```python
from build123d import *

# Parameters (mm, degrees)
BASE_FLANGE1_DEPTH = 1220
SKETCH6_W          = 10
SKETCH6_H          = 19.2634
CUT_EXTRUDE1_DEPTH = 1350.246604201
CUT_EXTRUDE2_REACH = 1300.516
FILLET1_R          = 1


# Sheet-metal steps are written as plain solids
with BuildPart() as part:
    # Sketch1 → Base-Flange1 (new body)
    with BuildSketch(Plane(origin=(0, 0, 0), x_dir=(0, 0, -1), z_dir=(1, 0, 0))):
        with BuildLine():
            Line((-128.767123288, 0.95890411), (-128.767123288, -13.30449589))
            ThreePointArc((-128.767123288, -13.30449589), (-128.551378143, -13.825350745), (-128.030523288, -14.04109589))
            Line((-128.030523288, -14.04109589), (440.496276712, -14.04109589))
            ThreePointArc((440.496276712, -14.04109589), (441.017131567, -13.825350745), (441.232876712, -13.30449589))
            Line((441.232876712, -13.30449589), (441.232876712, 5.95890411))
            Line((441.232876712, 5.95890411), (444.232876712, 5.95890411))
            Line((444.232876712, 5.95890411), (444.232876712, -13.30449589))
            ThreePointArc((444.232876712, -13.30449589), (443.138451911, -15.946671089), (440.496276712, -17.04109589))
            Line((440.496276712, -17.04109589), (-128.030523288, -17.04109589))
            ThreePointArc((-128.030523288, -17.04109589), (-130.672698486, -15.946671089), (-131.767123288, -13.30449589))
            Line((-131.767123288, -13.30449589), (-131.767123288, 0.95890411))
            Line((-131.767123288, 0.95890411), (-128.767123288, 0.95890411))
        make_face()
    extrude(amount=BASE_FLANGE1_DEPTH)

    # Sketch6 → Cut-Extrude1 (cut, through all)
    with BuildSketch(Plane(origin=(0, 0, -444.232876712), x_dir=(-1, 0, 0), z_dir=(0, 0, -1))):
        with Locations((-1215, -3.67279589)):
            Rectangle(SKETCH6_W, SKETCH6_H)
        with Locations((-5, -3.67279589)):
            Rectangle(SKETCH6_W, SKETCH6_H)
    extrude(amount=-CUT_EXTRUDE1_DEPTH, mode=Mode.SUBTRACT)

    # Sketch8 → Cut-Extrude2 (cut, up to next)
    with BuildSketch(Plane(origin=(0, -14.04109589, 0), x_dir=(1, 0, 0), z_dir=(0, 1, 0)), mode=Mode.PRIVATE) as cut_extrude2_sk1:
        with BuildLine():
            Line((903.689592114, 440.496276712), (783.689592114, 440.496276712))
            Line((783.689592114, 440.496276712), (783.689592114, 405.496276712))
            ThreePointArc((783.689592114, 405.496276712), (785.154058208, 401.960742806), (788.689592114, 400.496276712))
            Line((788.689592114, 400.496276712), (898.689592114, 400.496276712))
            ThreePointArc((898.689592114, 400.496276712), (902.22512602, 401.960742806), (903.689592114, 405.496276712))
            Line((903.689592114, 405.496276712), (903.689592114, 440.496276712))
        make_face()
    cut_extrude2_tool1 = extrude(cut_extrude2_sk1.sketch, amount=-CUT_EXTRUDE2_REACH, mode=Mode.PRIVATE) & part.part
    add(cut_extrude2_tool1.solids().sort_by_distance((843.689592, -14.041096, -420.538583))[0], mode=Mode.SUBTRACT)

    # Fillet1
    fillet1_edges = [part.edges().sort_by_distance(p)[0] for p in [
        (610, 5.95890411, -441.232876712),
        (610, 5.95890411, -444.232876712),
    ]]
    fillet(fillet1_edges, radius=FILLET1_R)


solid = part.part
```
Geometry: final body of the model. Coordinates: model frame, mm. A direction names the side the tool comes from. Coordinates: 2 decimals unless noted, no trailing zeros. Order: outer loops, then holes, each group sorted by start corner. A loop starts at its lowest first (then second) coordinate and runs counter-clockwise, first axis right, second up. Notation, with made-up numbers: M 29,19 L 36,19 A36 ccw 36,55 Z; hole C 56,20 d5. An arc over 180 degrees is marked long. Answer in a Markdown table with one row per item. Add a question column.
Q1. Contact query for flat-ended pins moving along their axis: P1, Ø3.5, axis at x = 1216, z = 130.5, coming from the +Y side; P2, Ø1.5, axis at y = -8.5, z = -442, coming from the -X side; P3, Ø1.5, axis at x = 870, y = -16, coming from the -Z side; P4, Ø1.5, axis at y = -12.5, z = -224.5, coming from the +X side. Output: stop coordinate, or through.
Q2. Section query D-D on x = 685.5. Return the cut outline in (y, z), and give its area (3 significant figures).
Q3. Reachability of faces 1 (the flat face through (601, -14.041, -152)), 2 (the flat face through (601, -17.041, -160)) from +Z, -Z, +X, -X, +Y, -Y: full face, straight path, thin tool, end or side. Return the list, or none.
Q4. Line query: L1, parallel to Z at x = 411.5, y = -9.25; L2, parallel to Z at x = 633, y = -13.5; L3, parallel to Y at x = 1103, z = -371.5. Output: solid intervals per line, ascending.
Q5. Section query B-B on y = -6. Return the cut outline in (x, z), and give its area (3 significant figures).
Q6. Section query C-C on z = -83.5. Return the cut outline in (x, y), and give its area (3 significant figures).
Q7. Section query A-A on x = 877. Return the cut outline in (y, z).
Completed:
| question | item | result |
|---|---|---|
| 1 | P1 | stops at y = -13.3 |
| 1 | P2 | stops at x = 10 |
| 1 | P3 | stops at z = -443.69 |
| 1 | P4 | passes through |
| 2 | outline | M -17.04,-440.5 A3.74 ccw -13.3,-444.23 L 4.96,-444.23 A1 ccw 5.96,-443.23 L 5.96,-442.23 A1 ccw 4.96,-441.23 L -13.3,-441.23 A0.74 cw -14.04,-440.5 L -14.04,128.03 A0.74 cw -13.3,128.77 L 0.96,128.77 L 0.96,131.77 L -13.3,131.77 A3.74 ccw -17.04,128.03 Z |
| 2 | area | 1,830 mm2 |
| 3 | face 1 | +X, -X, +Y |
| 3 | face 2 | +Z, -Z, +X, -X, -Y |
| 4 | L1 | z = -444.23 to -441.23, 128.77 to 131.77 |
| 4 | L2 | z = -444.23 to -441.21, 128.74 to 131.76 |
| 4 | L3 | y = -17.04 to -14.04 |
| 5 | outline | M 10,-444.23 L 1210,-444.23 L 1210,-441.23 L 10,-441.23 Z; M 10,128.77 L 1210,128.77 L 1210,131.77 L 10,131.77 Z |
| 5 | area | 7,200 mm2 |
| 6 | outline | M 0,-17.04 L 1220,-17.04 L 1220,-14.04 L 0,-14.04 Z |
| 6 | area | 3,660 mm2 |
| 7 | outline | M -17.04,-440.5 A3.74 ccw -13.3,-444.23 L 4.96,-444.23 A1 ccw 5.96,-443.23 L 5.96,-442.23 A1 ccw 4.96,-441.23 L -13.3,-441.23 A0.74 cw -14.04,-440.5 Z; M -17.04,-400.5 L -14.04,-400.5 L -14.04,128.03 A0.74 cw -13.3,128.77 L 0.96,128.77 L 0.96,131.77 L -13.3,131.77 A3.74 ccw -17.04,128.03 Z |
